from build123d import *

# Parameters (mm, degrees)
ESQUISSE1_W                     = 80
ESQUISSE1_H                     = 80
ESQUISSE1_R                     = 1.25
ESQUISSE1_R_2                   = 8
EXTRUSION1_DEPTH                = 5
ESQUISSE2_R                     = 1.25
ENL_V_MAT_EXTRU_1_DEPTH         = 57.789083458
R_P_TITION_LIN_AIRE1_COUNT      = 4
R_P_TITION_LIN_AIRE1_PITCH      = 20
R_P_TITION_LIN_AIRE1_COUNT_DIR2 = 4
R_P_TITION_LIN_AIRE1_PITCH_DIR2 = 20
CONG_1_R                        = 2


with BuildPart() as part:
    # Esquisse1 → Extrusion1 (new body)
    with BuildSketch(Plane(origin=(0, 0, 0), x_dir=(1, 0, 0), z_dir=(0, 1, 0))):
        Rectangle(ESQUISSE1_W, ESQUISSE1_H)
        with Locations(Location((-15, 15, 0), (0, 0, 270))):
            Circle(ESQUISSE1_R, mode=Mode.SUBTRACT)
        with Locations(Location((15, 15, 0), (0, 0, 90))):
            Circle(ESQUISSE1_R, mode=Mode.SUBTRACT)
        with Locations(Location((-15, -15, 0), (0, 0, 90))):
            Circle(ESQUISSE1_R, mode=Mode.SUBTRACT)
        with Locations(Location((15, -15, 0), (0, 0, 270))):
            Circle(ESQUISSE1_R, mode=Mode.SUBTRACT)
        with Locations(Location((-36, 36, 0), (0, 0, 270))):
            Circle(ESQUISSE1_R, mode=Mode.SUBTRACT)
        with Locations(Location((36, 36, 0), (0, 0, 90))):
            Circle(ESQUISSE1_R, mode=Mode.SUBTRACT)
        with Locations(Location((36, -36, 0), (0, 0, 270))):
            Circle(ESQUISSE1_R, mode=Mode.SUBTRACT)
        with Locations(Location((-36, -36, 0), (0, 0, 90))):
            Circle(ESQUISSE1_R, mode=Mode.SUBTRACT)
        with Locations(Location((0, 0, 0), (0, 0, 270))):
            Circle(ESQUISSE1_R_2, mode=Mode.SUBTRACT)
    extrude(amount=EXTRUSION1_DEPTH)

    # Esquisse2 → Enlèv. mat.-Extru.1 (cut, through all)
    with BuildSketch(Plane(origin=(0, 5, 0), x_dir=(1, 0, 0), z_dir=(0, 1, 0))):
        with Locations(Location((-30, 30, 0), (0, 0, 270))):
            Circle(ESQUISSE2_R)
    enl_v_mat_extru_1 = extrude(amount=-ENL_V_MAT_EXTRU_1_DEPTH, mode=Mode.SUBTRACT)

    # Répétition linéaire1: Enl_v. mat.-Extru.1 4 × 4, 4 skipped
    with Locations(*[(j * R_P_TITION_LIN_AIRE1_PITCH_DIR2, 0, i * R_P_TITION_LIN_AIRE1_PITCH) for i in range(R_P_TITION_LIN_AIRE1_COUNT) for j in range(R_P_TITION_LIN_AIRE1_COUNT_DIR2) if (i, j) not in ((0, 0), (1, 1), (1, 2), (2, 1), (2, 2))]):
        add(enl_v_mat_extru_1, mode=Mode.SUBTRACT)

    # Congé1
    cong_1_edges = [part.edges().sort_by_distance(p)[0] for p in [
        (-40, 2.5, -40),
        (40, 2.5, -40),
        (40, 2.5, 40),
        (-40, 2.5, 40),
    ]]
    fillet(cong_1_edges, radius=CONG_1_R)


solid = part.part
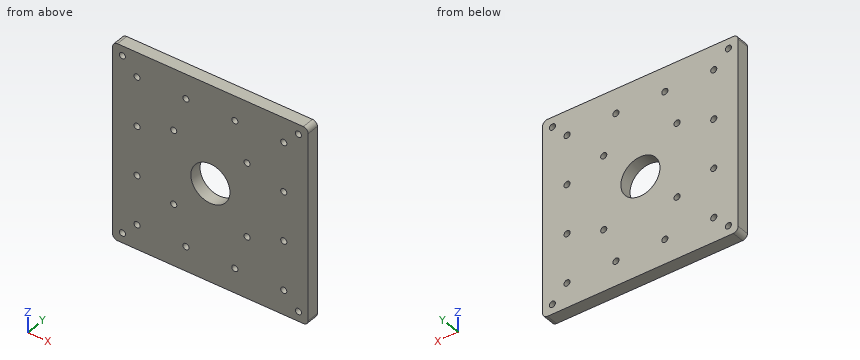
Geometry check sheet. Reference: the model listing, model coordinates, mm. Give positions to 0.01 mm unless a question says otherwise; leave off trailing zeros. Order: outer loops, then holes, each group sorted by start corner. A loop starts at its lowest first (then second) coordinate and runs counter-clockwise, first axis right, second up. Notation, with made-up numbers: (-36, 58) - (-11, 58) arc R23 ccw to (-11, 78) - close; hole circle Ø4 at (36, -15.75). An arc over 180 degrees is marked (long way). Use one line per item in the form item = value.
1) Sectioned sample at B-B (x = -36). Record the boundary of the cut face in (y, z), and give its area (3 significant figures).
Working result:
outline = (0, -40) - (5, -40) - (5, -37.25) - (0, -37.25) - close; (0, -34.75) - (5, -34.75) - (5, 34.75) - (0, 34.75) - close; (0, 37.25) - (5, 37.25) - (5, 40) - (0, 40) - close
area = 375 mm^2
2) Sectioned sample at A-A (x = 0). Record the boundary of the cut face in (y, z), and give its area (3 significant figures).
Working result:
outline = (0, -40) - (5, -40) - (5, -8) - (0, -8) - close; (0, 8) - (5, 8) - (5, 40) - (0, 40) - close
area = 320 mm^2
3) Sectioned sample at D-D (z = 3). Record the boundary of the cut face in (x, y), and give its area (3 significant figures).
Working result:
outline = (-40, 0) - (-7.42, 0) - (-7.42, 5) - (-40, 5) - close; (7.42, 0) - (40, 0) - (40, 5) - (7.42, 5) - close
area = 326 mm^2
4) Sectioned sample at C-C (y = 3.45). Count the separate pieces of the cut face and the enclosed holes in it, and give its area (3 significant figures).
Working result:
separate_pieces = 1
enclosed_holes = 21
area = 6,100 mm^2
5) Material ranges on probe 1 along X at (y, z) = (1.25, -30); probe 2 along X at (y, z) = (3.5, 36); probe 3 along X at (y, z) = (2.5, -10), recorded low to high. Write a range as from..to.
Working result:
probe_1 = -40..-31.25, -28.75..-11.25, -8.75..8.75, 11.25..28.75, 31.25..40
probe_2 = -40..-37.25, -34.75..34.75, 37.25..40
probe_3 = -40..-31.25, -28.75..28.75, 31.25..40
